Input: part model. Units: mm. Frame: model coordinates. A direction names the side the tool comes from. Coordinates: 2 decimals unless noted, no trailing zeros. Order: outer loops, then holes, each group sorted by start corner. A loop starts at its lowest first (then second) coordinate and runs counter-clockwise, first axis right, second up. Notation, with made-up numbers: M 18.25,-20 L 49.25,-20 A25 cw 49.25,2 Z; hole C 46,88 d8. An arc over 180 degrees is marked long. Answer in a Markdown table with one row per item.
from build123d import *

# Parameters (mm, degrees)
EXTRUDE_618_DEPTH   = 8
HOLE_WIZARD_M2_D    = 1.6
SKETCH_5_W          = 15
SKETCH_5_H          = 23
EXTRUDE_1905_DEPTH  = 8
FILLET_1_R          = 4
CUT_EXTRUDE_1_DEPTH = 60.03470161


with BuildPart() as part:
    # Эскиз1 → Extrude 618 (new body)
    with BuildSketch(Plane.XY):
        with BuildLine():
            Line((0.03033425, 5), (-14.96966575, 5))
            Line((-14.96966575, 5), (-14.96966575, 16.141238626))
            Line((-14.96966575, 16.141238626), (-38.828427125, 40))
            Line((-38.828427125, 40), (-39.64966575, 40))
            ThreePointArc((-39.64966575, 40), (-38.14966575, 41.5), (-39.64966575, 43))
            Line((-39.64966575, 43), (-34.757359313, 43))
            Line((-34.757359313, 43), (0.03033425, 8.212306438))
            Line((0.03033425, 8.212306438), (0.03033425, 5))
        make_face()
    extrude(amount=-EXTRUDE_618_DEPTH)

    # Крепление M2 (through all)
    with Locations(Plane.XY):
        with Locations((-2.96966575, 8), (-12.46966575, 17.5)):
            Hole(HOLE_WIZARD_M2_D / 2)

    # Эскиз5 → Extrude 1905 (add)
    with BuildSketch(Plane.XY):
        with Locations((-7.46966575, -6.5)):
            Rectangle(SKETCH_5_W, SKETCH_5_H)
    extrude(amount=-EXTRUDE_1905_DEPTH)

    # Скругление1
    # the kernel refuses this fillet: 4 mm, written as the material it adds along each edge
    with BuildSketch(Plane(origin=(-38.828427125, 40, 0), x_dir=(-1.0, -1.0209461682873532e-12, 0), z_dir=(0, 0, -1))) as fillet_1_piece_1:
        with BuildLine():
            CenterArc((1.771325284, -3.885528966), FILLET_1_R, 103.740313028, 31.259686972)
            Line((-1.057101841, -1.057101841), (0, 0))
            Line((0, 0), (0.821238626, 0))
        make_face()
    extrude(amount=8)
    with BuildSketch(Plane(origin=(-14.96966575, 16.141238626, 0), x_dir=(-0.7071067811865497, 0.7071067811865454, 0), z_dir=(0, 0, -1))) as fillet_1_piece_2:
        with BuildLine():
            CenterArc((FILLET_1_R * 0.414213562373, -FILLET_1_R), FILLET_1_R, 90, 45)
            Line((-FILLET_1_R * 0.292893218813, -FILLET_1_R * 0.292893218813), (0, 0))
            Line((0, 0), (FILLET_1_R * 0.414213562373, 0))
        make_face()
    extrude(amount=8)
    # the kernel refuses this fillet: 4 mm, written as the material it takes off along each edge
    with BuildSketch(Plane(origin=(-34.757359313, 43, 4.142135624), x_dir=(0.7071067811865497, -0.7071067811865454, 0), z_dir=(0, 0, -1)), Plane(origin=(0.03033425, 8.212306438, 4.142135624), x_dir=(0, -1, 0), z_dir=(0, 0, -1))) as fillet_1_2_piece_1:
        with BuildLine():
            CenterArc((FILLET_1_R * 0.414213562373, FILLET_1_R), FILLET_1_R, 225, 45)
            Line((-FILLET_1_R * 0.292893218813, FILLET_1_R * 0.292893218813), (0, 0))
            Line((0, 0), (FILLET_1_R * 0.414213562373, 0))
        make_face()
    extrude(amount=16.284271247, mode=Mode.SUBTRACT)
    with BuildSketch(Plane(origin=(-14.96966575, -18, 10), x_dir=(1, 0, 0), z_dir=(0, 0, -1))) as fillet_1_2_piece_2:
        with BuildLine():
            CenterArc((FILLET_1_R, -FILLET_1_R), FILLET_1_R, 90, 90)
            Line((0, -FILLET_1_R), (0, 0))
            Line((0, 0), (FILLET_1_R, 0))
        make_face()
    extrude(amount=28, mode=Mode.SUBTRACT)

    # Эскиз6 → Вырез-Вытянуть1 (cut, through all)
    with BuildSketch(Plane.XY):
        with BuildLine():
            Line((0.03033425, -6.540529805), (0.03033425, -19.459470195))
            ThreePointArc((0.03033425, -19.459470195), (-3.25, -13), (0.03033425, -6.540529805))
        make_face()
    extrude(amount=-CUT_EXTRUDE_1_DEPTH, mode=Mode.SUBTRACT)


solid = part.part
1) Cut plane C-C, the plane x = -22. Output: boundary loops of the cut face in (y, z).
Resolved:
| item | result |
|---|---|
| outline | M 23.17,-8 L 30.24,-8 L 30.24,0 L 23.17,0 Z |
2) Material intervals for probe 1 along X at (y, z) = (-1, -2.75); probe 2 along Y at (x, z) = (-12, -2.5); probe 3 along X at (y, z) = (26, -7), sorted ascending.
Resolved:
| item | result |
|---|---|
| probe 1 | x = -14.97 to 0.03 |
| probe 2 | y = -17.87 to 16.85, 18.15 to 20.24 |
| probe 3 | x = -24.83 to -17.76 |
3) Cut plane B-B, the plane z = -2.5. Output: boundary loops of the cut face in (x, y) (3 decimals), and give its area (3 significant figures).
Resolved:
| item | result |
|---|---|
| outline | M -39.65,40 A4 cw -37.771,38.943 L -16.141,17.313 A4 cw -14.97,14.484 L -14.97,-14 A4 ccw -10.97,-18 L -1.495,-18 A8 cw 0.03,-6.541 L 0.03,6.555 A4 ccw -1.141,9.384 L -33.586,41.828 A4 ccw -36.414,43 L -39.65,43 A1.5 cw Z; hole C -12.47,17.5 d1.6; hole C -2.97,8 d1.6 |
| area | 629 mm2 |
4) Reachability of faces 1 (the face through (-14.97, 0, -4)), 2 (the face through (-17.59, 25.83, -3.94)) from +Z, -Z, +X, -X, +Y, -Y: full face, straight path, thin tool, end or side. Return the list, or none.
Resolved:
| item | result |
|---|---|
| face 1 | +Z, -Z, -X, -Y |
| face 2 | +Z, -Z, +X, +Y |
5) Contact query for flat-ended pins moving along their axis: pin 1 (1.5 mm diameter, centred on y = 15, z = -2.5, fed in from -X); pin 2 (3 mm diameter, centred on y = 16.5, z = -6, fed in from -X); pin 3 (2.5 mm diameter, centred on x = -2.97, y = 8, fed in from -Z); pin 4 (4 mm diameter, centred on y = 24, z = -5, fed in from +X). Output: stop coordinate, or through.
Resolved:
| item | result |
|---|---|
| pin 1 | stops at x = -15.18 |
| pin 2 | stops at x = -16.83 |
| pin 3 | stops at z = -8 |
| pin 4 | stops at x = -13.76 |
6) Cut plane D-D, the plane y = -8.5. Output: boundary loops of the cut face in (x, z).
Resolved:
| item | result |
|---|---|
| outline | M -14.97,-8 L -1.86,-8 L -1.86,0 L -14.97,0 Z |
7) Cut plane A-A, the plane y = 8. Output: boundary loops of the cut face in (x, z), and give its area (3 significant figures).
Resolved:
| item | result |
|---|---|
| outline | M -14.97,-8 L -3.77,-8 L -3.77,0 L -14.97,0 Z; M -2.17,-8 L -0.24,-8 L -0.24,0 L -2.17,0 Z |
| area | 105 mm2 |
